from build123d import *

# Parameters (mm, degrees)
SKETCH1_R           = 3.175
SKETCH1_R_2         = 3.2639
SKETCH1_R_3         = 2.6289
SKETCH1_R_4         = 2.0193
BOSS_EXTRUDE1_DEPTH = 6.35
SKETCH2_R           = 3.175
CUT_EXTRUDE1_DEPTH  = 0.79375


with BuildPart() as part:
    # Sketch1 → Boss-Extrude1 (new body)
    with BuildSketch(Plane.XY):
        with BuildLine():
            Line((159.591131024, -50.8), (268.282803213, -50.8))
            ThreePointArc((268.282803213, -50.8), (272.859757692, 10.190933821), (263.746046868, 70.670540265))
            Line((263.746046868, 70.670540265), (234.864133392, 140.397647486))
            Line((234.864133392, 140.397647486), (234.123018172, 140.508771477))
            Line((234.123018172, 140.508771477), (152.715190262, 152.715190262))
            Line((152.715190262, 152.715190262), (118.427127597, 118.427127597))
            ThreePointArc((118.427127597, 118.427127597), (154.732498954, 64.092299607), (167.48125, 0))
            ThreePointArc((167.48125, 0), (165.496965553, -25.70454229), (159.591131024, -50.8))
        make_face()
        with Locations((176.898422575, 6.177429038)):
            Circle(SKETCH1_R, mode=Mode.SUBTRACT)
        with Locations((144.995031539, 101.526614087)):
            Circle(SKETCH1_R, mode=Mode.SUBTRACT)
        with Locations((163.532451502, 67.7373593)):
            Circle(SKETCH1_R, mode=Mode.SUBTRACT)
        with Locations((172.12665951, -41.275)):
            Circle(SKETCH1_R, mode=Mode.SUBTRACT)
        with Locations((193.675, 0)):
            Circle(SKETCH1_R_2, mode=Mode.SUBTRACT)
        with Locations((219.075, 0)):
            Circle(SKETCH1_R_2, mode=Mode.SUBTRACT)
        with Locations((215.746758491, 38.041974522)):
            Circle(SKETCH1_R_2, mode=Mode.SUBTRACT)
        with Locations((190.732641565, 33.63131081)):
            Circle(SKETCH1_R_2, mode=Mode.SUBTRACT)
        with Locations((205.863160899, 74.928062899)):
            Circle(SKETCH1_R_2, mode=Mode.SUBTRACT)
        with Locations((181.994968331, 66.240751259)):
            Circle(SKETCH1_R_2, mode=Mode.SUBTRACT)
        with Locations((189.724515334, 109.5375)):
            Circle(SKETCH1_R_2, mode=Mode.SUBTRACT)
        with Locations((167.727470078, 96.8375)):
            Circle(SKETCH1_R_2, mode=Mode.SUBTRACT)
        with Locations((167.821186376, 140.818695592)):
            Circle(SKETCH1_R_2, mode=Mode.SUBTRACT)
        with Locations((148.363657521, 124.491890306)):
            Circle(SKETCH1_R_2, mode=Mode.SUBTRACT)
        with Locations((263.525, 0)):
            Circle(SKETCH1_R_2, mode=Mode.SUBTRACT)
        with Locations((254.545603373, 68.205288861)):
            Circle(SKETCH1_R_2, mode=Mode.SUBTRACT)
        with Locations((228.219344532, 131.7625)):
            Circle(SKETCH1_R_2, mode=Mode.SUBTRACT)
        with Locations((177.875240911, 47.661527156)):
            Circle(SKETCH1_R_3, mode=Mode.SUBTRACT)
        with Locations((183.141207032, 19.248916511)):
            Circle(SKETCH1_R_3, mode=Mode.SUBTRACT)
        with Locations((139.323763183, 109.179217581)):
            Circle(SKETCH1_R_4, mode=Mode.SUBTRACT)
        with Locations((159.651941396, 76.436052669)):
            Circle(SKETCH1_R_4, mode=Mode.SUBTRACT)
        with Locations((176.974598028, -3.347266353)):
            Circle(SKETCH1_R_4, mode=Mode.SUBTRACT)
        with Locations((174.135237045, -31.751090662)):
            Circle(SKETCH1_R_4, mode=Mode.SUBTRACT)
        with Locations((240.38178065, 21.030680725)):
            Circle(SKETCH1_R_2, mode=Mode.SUBTRACT)
        with Locations((233.077901884, 62.453035583)):
            Circle(SKETCH1_R_2, mode=Mode.SUBTRACT)
        with Locations((218.692069012, 101.977786558)):
            Circle(SKETCH1_R_2, mode=Mode.SUBTRACT)
        with Locations((228.6, -38.1)):
            Circle(SKETCH1_R_3, mode=Mode.SUBTRACT)
        with Locations((254, -38.1)):
            Circle(SKETCH1_R_3, mode=Mode.SUBTRACT)
        with BuildLine():
            Line((202.565, 0), (202.565, 9.525))
            ThreePointArc((202.565, 9.525), (206.375, 13.335), (210.185, 9.525))
            Line((210.185, 9.525), (210.185, 0))
            Line((210.185, 0), (210.185, -9.525))
            ThreePointArc((210.185, -9.525), (206.375, -13.335), (202.565, -9.525))
            Line((202.565, -9.525), (202.565, 0))
        make_face(mode=Mode.SUBTRACT)
        with BuildLine():
            Line((199.487582489, 35.175043109), (201.141581381, 25.794749262))
            ThreePointArc((201.141581381, 25.794749262), (205.555298477, 22.70423128), (208.645816459, 27.117948375))
            Line((208.645816459, 27.117948375), (206.991817567, 36.498242223))
            Line((206.991817567, 36.498242223), (205.337818675, 45.87853607))
            ThreePointArc((205.337818675, 45.87853607), (200.924101579, 48.969054052), (197.833583597, 44.555336957))
            Line((197.833583597, 44.555336957), (199.487582489, 35.175043109))
        make_face(mode=Mode.SUBTRACT)
        with BuildLine():
            Line((190.348835729, 69.281310333), (193.606577595, 60.33073812))
            ThreePointArc((193.606577595, 60.33073812), (198.489903226, 58.053605981), (200.767035365, 62.936931612))
            Line((200.767035365, 62.936931612), (197.5092935, 71.887503825))
            Line((197.5092935, 71.887503825), (194.251551635, 80.838076038))
            ThreePointArc((194.251551635, 80.838076038), (189.368226003, 83.115208177), (187.091093864, 78.231882546))
            Line((187.091093864, 78.231882546), (190.348835729, 69.281310333))
        make_face(mode=Mode.SUBTRACT)
        with BuildLine():
            Line((175.426435918, 101.2825), (180.188935918, 93.033608029))
            ThreePointArc((180.188935918, 93.033608029), (185.393492706, 91.639051241), (186.788049494, 96.843608029))
            Line((186.788049494, 96.843608029), (182.025549494, 105.0925))
            Line((182.025549494, 105.0925), (177.263049494, 113.341391971))
            ThreePointArc((177.263049494, 113.341391971), (172.058492706, 114.735948759), (170.663935918, 109.531391971))
            Line((170.663935918, 109.531391971), (175.426435918, 101.2825))
        make_face(mode=Mode.SUBTRACT)
        with BuildLine():
            Line((155.17379262, 130.206272156), (161.296344603, 122.909698835))
            ThreePointArc((161.296344603, 122.909698835), (166.663994724, 122.4400903), (167.133603259, 127.807740421))
            Line((167.133603259, 127.807740421), (161.011051277, 135.104313742))
            Line((161.011051277, 135.104313742), (154.888499295, 142.400887063))
            ThreePointArc((154.888499295, 142.400887063), (149.520849174, 142.870495598), (149.051240638, 137.502845477))
            Line((149.051240638, 137.502845477), (155.17379262, 130.206272156))
        make_face(mode=Mode.SUBTRACT)
    extrude(amount=BOSS_EXTRUDE1_DEPTH)

    # Sketch2 → Cut-Extrude1 (cut)
    with BuildSketch(Plane.XY):
        with Locations((202.565, 0)):
            Circle(SKETCH2_R)
        with Locations((210.185, 0)):
            Circle(SKETCH2_R)
        with Locations((199.487582489, 35.175043109)):
            Circle(SKETCH2_R)
        with Locations((206.991817567, 36.498242223)):
            Circle(SKETCH2_R)
        with Locations((190.348835729, 69.281310333)):
            Circle(SKETCH2_R)
        with Locations((197.5092935, 71.887503825)):
            Circle(SKETCH2_R)
        with Locations((175.426435918, 101.2825)):
            Circle(SKETCH2_R)
        with Locations((182.025549494, 105.0925)):
            Circle(SKETCH2_R)
        with Locations((155.17379262, 130.206272156)):
            Circle(SKETCH2_R)
        with Locations((161.011051277, 135.104313742)):
            Circle(SKETCH2_R)
    extrude(amount=CUT_EXTRUDE1_DEPTH, mode=Mode.SUBTRACT)


solid = part.part
Source: CAD feature listing. Evaluate the final solid. Frame: model axes, mm. A direction names the side the tool comes from. Round coordinates to 2 decimals unless told otherwise and drop trailing zeros. Loops run counter-clockwise (first coordinate to the right, second up) from the corner with the lowest first, then second, coordinate; pieces in that order, holes last. Notation, with made-up numbers: (85.25, 49) - (98.25, 49) arc R24 cw to (98.25, 63) - close; hole circle Ø9 at (14.25, -22.75). An arc over 180 degrees is marked (long way). Write item = value, one per line. Start each with the question number.
Item 1: Material intervals for line 1 (X direction, y = 94, z = 0.75); line 2 (X direction, y = 7.5, z = 5.5) (3 decimals); line 3 (Y direction, x = 203, z = 3.5), sorted ascending.
Item 2: Section query B-B on y = -18. Output: boundary loops of the cut face in (x, z), plus the area to 3 significant figures.
Item 3: Section query A-A on x = 254. Output: boundary loops of the cut face in (y, z).
Item 4: Section query C-C on z = 2. Count the separate pieces of the cut face and the enclosed holes in it, plus the area to 3 significant figures.
Item 5: First-contact query: pin 1 Ø2 at (x, z) = (220, 1.5) entering from +Y; pin 2 Ø1.1 at (x, y) = (198, 34.5) entering from -Z; pin 3 Ø1 at (y, z) = (46.5, 1.5) entering from -X. Flat tips, straight axial feed; report the tip coordinate or a pass-through.
Item 6: Mould query, pull axis X, two halves, no side actions, for faces 4 (the face through (272.89, 9.33, 3.13)), 5 (the face through (212, 52, 0)), 6 (the face through (213.157, 36.056, 3.131)). Classes: released by +X, released by -X, zero draft, split by the parting line, or undercut.
Item 7: Reachability of faces 1 (the face through (136, 136, 3)), 2 (the face through (175.36, 101.4, 3.13)), 3 (the face through (174, 100, 0.794)) from +Z, -Z, +X, -X, +Y, -Y: full face, straight path, thin tool, end or side. Return the list, or none.
Results list:
q1.line_1 = 138.61 to 166.11, 169.34 to 179.63, 187.18 to 254.08
q1.line_2 = 167.313 to 174.012, 179.785 to 202.565, 210.185 to 272.947
q1.line_3 = -50.8 to -11.29, 11.29 to 23.15, 48.75 to 73.36, 76.5 to 145.18
q2.outline = (166.51, 0) - (272.46, 0) - (272.46, 6.35) - (166.51, 6.35) - close
q2.area = 673 mm²
q3.outline = (-50.8, 0) - (-40.73, 0) - (-40.73, 6.35) - (-50.8, 6.35) - close; (-35.47, 0) - (64.99, 0) - (64.99, 6.35) - (-35.47, 6.35) - close; (71.42, 0) - (94.2, 0) - (94.2, 6.35) - (71.42, 6.35) - close
q4.separate_pieces = 1
q4.enclosed_holes = 33
q4.area = 19,800 mm²
q5.pin_1 = 142.78
q5.pin_2 = 0.79
q5.pin_3 = 160.75
q6.face_4 = released by +X
q6.face_5 = zero draft
q6.face_6 = undercut
q7.face_1 = +Z, -Z, -X, +Y
q7.face_2 = +Z, -Z
q7.face_3 = -Z
